from build123d import *

# Parameters (mm, degrees)
SKETCH_1_W               = 20
SKETCH_1_H               = 12
SKETCH_1_R               = 2
EXTRUDE_1_DEPTH          = 5
CUT_EXTRUDE_1_DEPTH      = 13.68857754
CUT_EXTRUDE_1_DEPTH_BACK = 13.68857754
SKETCH_2_R               = 2


with BuildPart() as part:
    # 草图1 → 凸台-拉伸1 (new, symmetric)
    with BuildSketch(Plane(origin=(0, 0, 0), x_dir=(1, 0, 0), z_dir=(0, 1, 0))):
        Rectangle(SKETCH_1_W, SKETCH_1_H)
        with Locations(Location((0, -2, 0), (0, 0, 270))):
            Circle(SKETCH_1_R, mode=Mode.SUBTRACT)
    extrude(amount=EXTRUDE_1_DEPTH, both=True)

    # 草图2 → 切除-拉伸1 (cut, two sides: drawn at the far end of the back side and taken through both)
    with BuildSketch(Plane.XY.offset(-CUT_EXTRUDE_1_DEPTH_BACK)):
        with Locations((-5, 0)):
            Circle(SKETCH_2_R)
        with Locations(Location((5, 0, 0), (0, 0, 180))):
            Circle(SKETCH_2_R)
    extrude(amount=CUT_EXTRUDE_1_DEPTH + CUT_EXTRUDE_1_DEPTH_BACK, mode=Mode.SUBTRACT)


solid = part.part
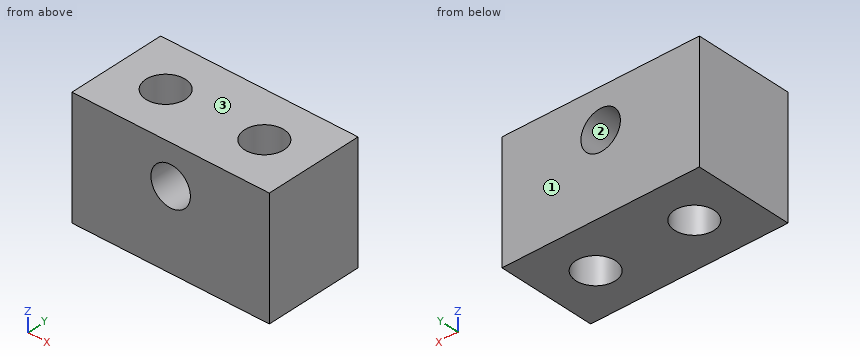
Verification items for the finished model (mm, model axes). Face numbers are marked on the shaded views. Round coordinates to 2 decimals unless told otherwise and drop trailing zeros. Loops run counter-clockwise (first coordinate to the right, second up) from the corner with the lowest first, then second, coordinate; pieces in that order, holes last. Notation, with made-up numbers: (21.25, 43) - (79.25, 43) arc R20 ccw to (79.25, 66) - close; hole circle Ø10 at (-5.5, -22.75). An arc over 180 degrees is marked (long way). Answer in a Markdown table with one row per item. Add a question column.
Q1. Section check D-D on z = -1.75. Enter the section's corners in (x, y).
Q2. Gauge pin test, flat ends, axial feed: pin 1 (4.5 mm diameter, centred on x = -5, y = 0, fed in from -Z); pin 2 (3.5 mm diameter, centred on x = 0, z = 2, fed in from +Y). Record the tip position at first contact, or that the pin passes through.
Q3. Section check B-B on x = 5. Enter the section's corners in (y, z).
Q4. Release check for a two-part mould opening along Z. For the marked faces 1, 2 and 3 record: pulls with the +Z half, pulls with the -Z half, needs draft (parallel to the pull), parting line crosses it, or undercut.
Q5. Material ranges on line 1 (Y direction, x = 5, z = 4); line 2 (X direction, y = -1.25, z = -1.25); line 3 (X direction, y = 0.25, z = 2), recorded low to high.
Q6. Section check A-A on z = 2. Enter the section's corners in (x, y).
Q7. Section check C-C on y = 0. Enter the section's corners in (x, z), plus the area to 3 significant figures.
Found:
| question | item | result |
|---|---|---|
| 1 | outline | (-10, -5) - (10, -5) - (10, 5) - (-10, 5) - close; hole circle Ø4 at (-5, 0); hole circle Ø4 at (5, 0) |
| 2 | pin 1 | stops at z = -6 |
| 2 | pin 2 | passes through |
| 3 | outline | (-5, -6) - (-2, -6) - (-2, 6) - (-5, 6) - close; (2, -6) - (5, -6) - (5, 6) - (2, 6) - close |
| 4 | face 1 | needs draft |
| 4 | face 2 | undercut |
| 4 | face 3 | pulls with the +Z half |
| 5 | line 1 | y = -5 to -2, 2 to 5 |
| 5 | line 2 | x = -10 to -6.56, -3.44 to 3.44, 6.56 to 10 |
| 5 | line 3 | x = -10 to -6.98, -3.02 to -2, 2 to 3.02, 6.98 to 10 |
| 6 | outline | (-10, -5) - (-2, -5) - (-2, 5) - (-10, 5) - close; (2, -5) - (10, -5) - (10, 5) - (2, 5) - close; hole circle Ø4 at (-5, 0); hole circle Ø4 at (5, 0) |
| 7 | outline | (-10, -6) - (-7, -6) - (-7, 6) - (-10, 6) - close; (-3, -6) - (3, -6) - (3, 6) - (-3, 6) - close; (7, -6) - (10, -6) - (10, 6) - (7, 6) - close; hole circle Ø4 at (0, 2) |
| 7 | area | 131 mm² |
